from build123d import *

# Parameters (mm, degrees)
SKETCH1_W           = 25.4
SKETCH1_H           = 12.7
BOSS_EXTRUDE1_DEPTH = 6.985
SKETCH3_W           = 3.175
SKETCH3_H           = 12.7
BOSS_EXTRUDE2_DEPTH = 15.875
SKETCH4_W           = 3.175
SKETCH4_H           = 12.7
BOSS_EXTRUDE3_DEPTH = 15.875
SKETCH5_R           = 1.5875
CUT_EXTRUDE2_DEPTH  = 33.50927137
SKETCH6_R           = 3.81
CUT_EXTRUDE3_DEPTH  = 35.757187746
SKETCH7_R           = 1.5875
CUT_EXTRUDE4_DEPTH  = 34.050514746


with BuildPart() as part:
    # Sketch1 → Boss-Extrude1 (new, symmetric)
    with BuildSketch(Plane.XY):
        Rectangle(SKETCH1_W, SKETCH1_H)
    extrude(amount=BOSS_EXTRUDE1_DEPTH, both=True)

    # Sketch3 → Boss-Extrude2 (add)
    with BuildSketch(Plane(origin=(0, 0, -6.985), x_dir=(-1, 0, 0), z_dir=(0, 0, -1))):
        with Locations((-11.1125, 0)):
            Rectangle(SKETCH3_W, SKETCH3_H)
    extrude(amount=BOSS_EXTRUDE2_DEPTH)

    # Sketch4 → Boss-Extrude3 (add)
    with BuildSketch(Plane.XY.offset(6.985)):
        with Locations((11.1125, 0)):
            Rectangle(SKETCH4_W, SKETCH4_H)
    extrude(amount=BOSS_EXTRUDE3_DEPTH)

    # Sketch5 → Cut-Extrude2 (cut, through all)
    with BuildSketch(Plane.ZY.offset(-9.525)):
        with Locations(Location((-20.32, 0, 0), (0, 0, 270))):
            Circle(SKETCH5_R)
        with Locations(Location((20.32, 0, 0), (0, 0, 270))):
            Circle(SKETCH5_R)
    extrude(amount=-CUT_EXTRUDE2_DEPTH, mode=Mode.SUBTRACT)

    # Sketch6 → Cut-Extrude3 (cut, through all)
    with BuildSketch(Plane.ZY.offset(12.7)):
        Circle(SKETCH6_R)
    extrude(amount=-CUT_EXTRUDE3_DEPTH, mode=Mode.SUBTRACT)

    # Sketch7 → Cut-Extrude4 (cut, through all)
    with BuildSketch(Plane.XY.offset(6.985)):
        with Locations((-6.20047096, 0)):
            Circle(SKETCH7_R)
    extrude(amount=-CUT_EXTRUDE4_DEPTH, mode=Mode.SUBTRACT)


solid = part.part
Verification items for the finished model (mm, model axes). A direction names the side the tool comes from. Coordinates: 2 decimals unless noted, no trailing zeros. Order: outer loops, then holes, each group sorted by start corner. A loop starts at its lowest first (then second) coordinate and runs counter-clockwise, first axis right, second up. Notation, with made-up numbers: (78, 62.5) -> (111, 62.5) arc R21 cw to (111, 66.5) -> close; hole circle Ø11 at (-21.5, -21). An arc over 180 degrees is marked (long way). Use CSV: the item, a comma, the result in double quotes. Start each with the question number.
Q1. Section check C-C, the plane x = -8.75. Record the cut outline in (y, z) (3 decimals).
Q2. Thickness scan on line 1 along Z through (x, y) = (11.5, 0); line 2 along Z through (x, y) = (2.5, 0) (3 decimals); line 3 along X through (y, z) = (0, 5.55). Record the ranges inside material, lowest first.
Q3. Draft check along Y on faces 4 (the flat face through (3, 6.35, 0)), 5 (the cylindrical face through (11.09, 0.207, -18.746)), 6 (the flat face through (9.525, 0, -15)), 7 (the flat face through (3, -6.35, 0)). Enter one of: +Y half, -Y half, draft (parallel to the pull), parting line (faces both ways), or undercut.
Q4. Depth check by flat-ended pin: P1, Ø3, axis at y = 0, z = -20.32, coming from the -X side; P2, Ø6.5, axis at x = -5.5, y = 3, coming from the +Z side (3 decimals); P3, Ø6.5, axis at y = 2, z = 17.5, coming from the -X side (3 decimals); P4, Ø1, axis at x = 8, y = 4, coming from the -Z side (3 decimals). Enter the tip coordinate at first touch or a pass-through.
Q5. Tool access check on faces 1 (the flat face through (-2, 0, -6.985)), 2 (the flat face through (12.7, 4, 0)), 3 (the flat face through (-2, 0, 6.985)). Record the directions out of +Z, -Z, +X, -X, +Y, -Y that give a thin tool (end or side, any length) a straight path to the whole face; none if there is none.
Q6. Section check B-B, the plane y = 0. Record the cut outline in (x, z) (1 decimal).
Returned:
1,outline,"(-6.35, -6.985) -> (6.35, -6.985) -> (6.35, 6.985) -> (-6.35, 6.985) -> close; hole circle Ø7.62 at (0, 0)"
2,line 1,"z = -22.86 to -21.91, -18.73 to -3.81, 3.81 to 18.73, 21.91 to 22.86"
2,line 2,"z = -6.985 to -3.81, 3.81 to 6.985"
2,line 3,"x = -12.7 to -7.79, -4.61 to 12.7"
3,face 4,"+Y half"
3,face 5,"undercut"
3,face 6,"draft"
3,face 7,"-Y half"
4,P1,"passes through"
4,P2,"stops at z = 6.985"
4,P3,"stops at x = 9.525"
4,P4,"stops at z = -6.985"
5,face 1,"-Z, -X, +Y, -Y"
5,face 2,"+Z, -Z, +X, +Y, -Y"
5,face 3,"+Z, -X, +Y, -Y"
6,outline,"(-12.7, -7) -> (-7.8, -7) -> (-7.8, -3.8) -> (-12.7, -3.8) -> close; (-12.7, 3.8) -> (-7.8, 3.8) -> (-7.8, 7) -> (-12.7, 7) -> close; (-4.6, -7) -> (9.5, -7) -> (9.5, -18.7) -> (12.7, -18.7) -> (12.7, -3.8) -> (-4.6, -3.8) -> close; (-4.6, 3.8) -> (12.7, 3.8) -> (12.7, 18.7) -> (9.5, 18.7) -> (9.5, 7) -> (-4.6, 7) -> close; (9.5, -22.9) -> (12.7, -22.9) -> (12.7, -21.9) -> (9.5, -21.9) -> close; (9.5, 21.9) -> (12.7, 21.9) -> (12.7, 22.9) -> (9.5, 22.9) -> close"
